Part model, mm, in its own coordinate system. Give positions to 0.01 mm unless a question says otherwise; leave off trailing zeros. Order: outer loops, then holes, each group sorted by start corner. A loop starts at its lowest first (then second) coordinate and runs counter-clockwise, first axis right, second up. Notation, with made-up numbers: M 50.25,-26.75 L 78.25,-26.75 A23 ccw 78.25,11.25 Z; hole C 88,56 d5. An arc over 180 degrees is marked long. Return JSON: item names as keys, results as strings.
Autodesk Inventor part; units mm, degrees
ref_plane "YZ Plane" through (0, 0, 0) normal (1, 0, 0) x (0, 1, 0)
ref_plane "XZ Plane" through (0, 0, 0) normal (0, 1, 0) x (-1, 0, 0)
ref_plane "XY Plane" through (0, 0, 0) normal (0, 0, 1) x (1, 0, 0)
sketch "Skizze1" plane through (0, 0, 0) normal (0, 1, 0) x (-1, 0, 0)
  circle A0 centre (0, 0) radius 15
  circle A1 centre (0, 0) radius 6
  circle A2 centre (0, 0) radius 11
  line L0 (0, 0) -> (-26.7883, 0)
  line L1 (0, 0) -> (13.3942, -23.1994)
  line L2 (0, 0) -> (13.3942, 23.1994)
  circle A3 centre (5.5, -9.5263) radius 1.6
  circle A4 centre (5.5, 9.5263) radius 1.6
  circle A5 centre (-11, 0) radius 1.6
  dimension "d0" = 30
  dimension "d1" = 12
  dimension "d3" = 22
  dimension "d6" = 360
  dimension "d8" = 3.2
  dimension "d9" = 3.2
  dimension "d10" = 3.2
extrude "Extrusion1" add sketch "Skizze1" along normal blind 4 contours A0 L1 A3 A2 A4 L2 | L2 A4 A2 A5 L0 A0 | A0 L0 A5 A2 A3 L1 | A4 L2 A1 L0 A5 A2 | A2 A5 L0 A1 L1 A3 | A2 A3 L1 A1 L2 A4
properties part number "01-03-01-02 Zeichnung Zange links oben"
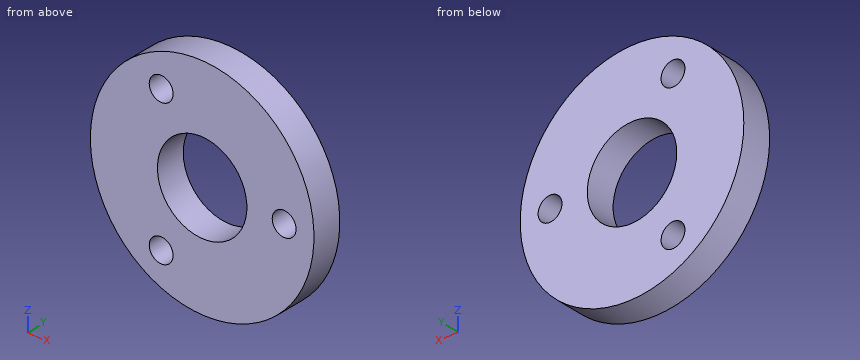
Q1. Band-saw the part on D-D (y = 3.35). Give the cut face in (x, z).
Established:
{"outline": "C 0,0 d30; hole C -5.5,-9.53 d3.2; hole C -5.5,9.53 d3.2; hole C 0,0 d12; hole C 11,0 d3.2"}
Q2. Band-saw the part on B-B (x = -5.5). Give the cut face in (y, z), then the cut area to 3 significant figures.
Established:
{"outline": "M 0,-13.96 L 4,-13.96 L 4,-11.13 L 0,-11.13 Z; M 0,-7.93 L 4,-7.93 L 4,-2.4 L 0,-2.4 Z; M 0,2.4 L 4,2.4 L 4,7.93 L 0,7.93 Z; M 0,11.13 L 4,11.13 L 4,13.96 L 0,13.96 Z", "area": "66.9 mm²"}
Q3. Band-saw the part on C-C (z = 4). Give the cut face in (x, y).
Established:
{"outline": "M -14.46,0 L -4.47,0 L -4.47,4 L -14.46,4 Z; M 4.47,0 L 14.46,0 L 14.46,4 L 4.47,4 Z"}
Q4. Pin check, flat tips, straight feed: pin 1 (7 mm diameter, centred on x = 0, z = 0, fed in from -Y); pin 2 (4 mm diameter, centred on x = -10, z = 7, fed in from -Y). Stop position of each tip, or through.
Established:
{"pin 1": "passes through", "pin 2": "stops at y = 0"}
Q5. Probe line 1 along Z through (x, y) = (-5.5, 3.1); line 2 along Z through (x, y) = (0, 1.4); line 3 along X through (y, z) = (1, 0). List the from-to ranges inside material, lowest first.
Established:
{"line 1": "z = -13.96 to -11.13, -7.93 to -2.4, 2.4 to 7.93, 11.13 to 13.96", "line 2": "z = -15 to -6, 6 to 15", "line 3": "x = -15 to -6, 6 to 9.4, 12.6 to 15"}
Q6. Band-saw the part on A-A (x = 0). Give the cut face in (y, z).
Established:
{"outline": "M 0,-15 L 4,-15 L 4,-6 L 0,-6 Z; M 0,6 L 4,6 L 4,15 L 0,15 Z"}
